Geometry: final body of the model. Coordinates: model frame, mm. A direction names the side the tool comes from. Give positions to 0.01 mm unless a question says otherwise; leave off trailing zeros. Order: outer loops, then holes, each group sorted by start corner. A loop starts at its lowest first (then second) coordinate and runs counter-clockwise, first axis right, second up. Notation, with made-up numbers: M 25,35 L 38,35 A14 ccw 38,41 Z; hole C 1,17 d2. An arc over 180 degrees is marked long. One line per item, written item: value. Start each with the question number.
```python
from build123d import *

# Parameters (mm, degrees)
F3_DEPTH = 1
F4_R     = 1.5
F5_DEPTH = 4.5
F6_R     = 0.5


with BuildPart() as f3:
    # F2 (on Top) → F3 (new body)
    with BuildSketch(Plane.XY):
        with BuildLine():
            Line((17.1622320903, 13.4306918032), (4.9303248829, 3.8583369368))
            ThreePointArc((4.9303248829, 3.8583369368), (0, 2.1584874548), (-4.9303248829, 3.8583369368))
            Line((-4.9303248829, 3.8583369368), (-17.1622320903, 13.4306918032))
            ThreePointArc((-17.1622320903, 13.4306918032), (-17.376145966, 13.4514618026), (-17.4853738885, 13.2663677724))
            Line((-17.4853738885, 13.2663677724), (-16.7529162453, -8.1999925091))
            ThreePointArc((-16.7529162453, -8.1999925091), (-16.6546778346, -8.3654169511), (-16.4623768157, -8.3714460037))
            Line((-16.4623768157, -8.3714460037), (-3.6262301421, -1.8440101433))
            ThreePointArc((-3.6262301421, -1.8440101433), (0, -0.9749606379), (3.6262301421, -1.8440101433))
            Line((3.6262301421, -1.8440101433), (16.4623768157, -8.3714460037))
            ThreePointArc((16.4623768157, -8.3714460037), (16.6546778346, -8.3654169511), (16.7529162453, -8.1999925091))
            Line((16.7529162453, -8.1999925091), (17.4853738885, 13.2663677724))
            ThreePointArc((17.4853738885, 13.2663677724), (17.376145966, 13.4514618026), (17.1622320903, 13.4306918032))
        make_face()
    extrude(amount=F3_DEPTH)

    # F4 (on face) → F5 (join)
    with BuildSketch(Plane.XY.offset(1)):
        with Locations((0, 0.5917634084)):
            Circle(F4_R)
    extrude(amount=F5_DEPTH)

    # F6
    f6_edges = [f3.edges().sort_by_distance(p)[0] for p in [
        (-1.5, 0.591763, 5.5),
    ]]
    fillet(f6_edges, radius=F6_R)


solid = f3.part
```
Q1. Section query D-D on z = 1.55. Return loops of the section in (x, y), and give its area (3 significant figures).
Q2. Ray query, line 1 along Z through (x, y) = (11, 8.25); line 2 along X through (y, z) = (-2, 0.55); line 3 along X through (y, z) = (0.25, 3.25). Return the intervals inside material, ascending. Write a range as [from, to].
Q3. Section query B-B on x = 0. Return loops of the section in (y, z), and give its area (3 significant figures).
Q4. Set-up query: faces 4 (the face through (9.95, -5.06, 0.49)), 5 (the face through (-10.961, 8.578, 0.493)), 6 (the face through (0, 1, 5.5)). Return all of +Z, -Z, +X, -X, +Y, -Y with unobstructed straight access to the full face (end or side cutting, diameter ignored); none if empty.
Q5. Mould query, pull axis X, two halves, no side actions, for faces 1 (the face through (-0.33, -0.87, 2.97)), 2 (the face through (0, 0, 0)), 3 (the face through (11.13, 8.71, 0.49)). Classes: +X half, -X half, draft (parallel to the pull), parting line (faces both ways), or undercut.
Q6. Section query C-C on y = -5. Return loops of the section in (x, z), and give its area (3 significant figures).
Q7. Contact query for flat-ended pins moving along their axis: pin 1 (3 mm diameter, centred on y = 1.5, z = 3, fed in from +X); pin 2 (1.5 mm diameter, centred on y = 6.5, z = 3, fed in from -X); pin 3 (6 mm diameter, centred on x = 12, y = -1.5, fed in from +Z); pin 4 (2 mm diameter, centred on x = 0, z = 5, fed in from +Y). Output: stop coordinate, or through.
Q8. Section query A-A on y = -1.5. Return loops of the section in (x, z), and give its area (3 significant figures).
Results below:
1. outline: C 0,0.59 d3
1. area: 7.07 mm2
2. line 1: [0, 1]
2. line 2: [-16.96, -3.93], [3.93, 16.96]
2. line 3: [-1.46, 1.46]
3. outline: M -0.97,0 L 2.16,0 L 2.16,1 L 2.09,1 L 2.09,5 A0.5 ccw 1.59,5.5 L -0.41,5.5 A0.5 ccw -0.91,5 L -0.91,1 L -0.97,1 Z
3. area: 16.5 mm2
4. face 4: +Z, -Z, -Y
4. face 5: +Z, -Z, +Y
4. face 6: +Z, +X, -X, +Y, -Y
5. face 1: parting line
5. face 2: draft
5. face 3: undercut
6. outline: M -16.86,0 L -9.83,0 L -9.83,1 L -16.86,1 Z; M 9.83,0 L 16.86,0 L 16.86,1 L 9.83,1 Z
6. area: 14.1 mm2
7. pin 1: x = 1.5
7. pin 2: through
7. pin 3: z = 1
7. pin 4: y = 2.09
8. outline: M -16.98,0 L -2.85,0 L -2.85,1 L -16.98,1 Z; M 2.85,0 L 16.98,0 L 16.98,1 L 2.85,1 Z
8. area: 28.3 mm2
